For this review, take the finished solid that the model builds, in its own axes (mm). A direction names the side the tool comes from. Give positions to 0.01 mm unless a question says otherwise; leave off trailing zeros. Loops run counter-clockwise (first coordinate to the right, second up) from the corner with the lowest first, then second, coordinate; pieces in that order, holes last. Notation, with made-up numbers: (56.25, 18.5) - (109.25, 18.5) arc R18 cw to (109.25, 38.5) - close; hole circle Ø1 at (54, -10.5). An arc over 180 degrees is marked (long way). Answer in a Markdown table with one row per item.
```python
from build123d import *

# Parameters (mm, degrees)
F0_W      = 30
F0_H      = 43
F1_DEPTH  = 10
F2_W      = 20
F2_H      = 10
F3_DEPTH  = 15
F5_D      = 5.5
F7_D      = 9
F7_DEPTH  = 5
F7_TIP    = 2.7038727856
F8_W      = 20
F8_H      = 43
F9_DEPTH  = 1.55
F11_D     = 3.3
F13_D     = 6
F13_DEPTH = 3
F13_TIP   = 1.8025818571
F14_W     = 6.5
F14_H     = 10
F15_DEPTH = 3.2
F17_D     = 11
F17_DEPTH = 3.5
F17_TIP   = 3.3047334047
F18_R     = 2


with BuildPart() as f1:
    # F0 (on Front) → F1 (new body)
    with BuildSketch(Plane.XZ):
        Rectangle(F0_W, F0_H)
    extrude(amount=F1_DEPTH)

    # F2 (on face) → F3 (join)
    with BuildSketch(Plane.XZ.offset(10)):
        with Locations((0, -16.5)):
            Rectangle(F2_W, F2_H)
    extrude(amount=F3_DEPTH)

    # F5 (through all)
    with Locations(Plane.XY.offset(-11.5)):
        with Locations((0, -17.5)):
            Hole(F5_D / 2)

    # F7
    with Locations(Plane.XY.offset(-11.5)):
        with Locations((0, -17.5)):
            Hole(F7_D / 2, depth=F7_DEPTH)
            with Locations((0, 0, -(F7_DEPTH + F7_TIP / 2))):  # 118° drill point
                Cone(0, F7_D / 2, F7_TIP, mode=Mode.SUBTRACT)

    # F8 (on face) → F9 (cut)
    with BuildSketch(Plane(origin=(0, 0, 0), x_dir=(-1, 0, 0), z_dir=(0, 1, 0))):
        Rectangle(F8_W, F8_H)
    extrude(amount=-F9_DEPTH, mode=Mode.SUBTRACT)

    # F11 (through all)
    with Locations(Plane(origin=(0, -1.55, 0), x_dir=(-1, 0, 0), z_dir=(0, 1, 0))):
        with Locations((0, 1.5)):
            Hole(F11_D / 2)

    # F13
    with Locations(Plane.XZ.offset(10)):
        with Locations((0, 1.5)):
            Hole(F13_D / 2, depth=F13_DEPTH)
            with Locations((0, 0, -(F13_DEPTH + F13_TIP / 2))):  # 118° drill point
                Cone(0, F13_D / 2, F13_TIP, mode=Mode.SUBTRACT)

    # F14 (on face) → F15 (cut)
    with BuildSketch(Plane(origin=(0, -1.55, 0), x_dir=(-1, 0, 0), z_dir=(0, 1, 0))):
        with Locations((-4.25, 16.5)):
            Rectangle(F14_W, F14_H)
        with Locations((-4.25, -16.5)):
            Rectangle(F14_W, F14_H)
    extrude(amount=-F15_DEPTH, mode=Mode.SUBTRACT)

    # F17
    with Locations(Plane(origin=(0, -1.55, 0), x_dir=(-1, 0, 0), z_dir=(0, 1, 0))):
        with Locations((-4.25, -8.5), (-4.25, 11.5)):
            Hole(F17_D / 2, depth=F17_DEPTH)
            with Locations((0, 0, -(F17_DEPTH + F17_TIP / 2))):  # 118° drill point
                Cone(0, F17_D / 2, F17_TIP, mode=Mode.SUBTRACT)

    # F18
    f18_edges = [f1.edges().sort_by_distance(p)[0] for p in [
        (-15, -5, 21.5),
        (0, -10, 21.5),
        (-15, -10, 0),
        (15, -5, 21.5),
        (15, -10, 0),
    ]]
    fillet(f18_edges, radius=F18_R)


solid = f1.part
```
1. We need section D-D, the plane y = -9. Give the boundary of the cut face in (x, z).
Values:
| item | result |
|---|---|
| outline | (-14.73, -21.5) - (14.73, -21.5) - (14.73, 19.5) arc R1.73 ccw to (13, 21.23) - (-13, 21.23) arc R1.73 ccw to (-14.73, 19.5) - close; hole circle Ø6 at (0, 1.5) |
2. Wall thickness on line 1 (X direction, y = -17.5, z = -13.85); line 2 (Z direction, x = 0, y = -3); line 3 (X direction, y = -3, z = 11.5): over which ranges is each line inside the solid? List them lowest first. Write a range as [from, to].
Values:
| item | result |
|---|---|
| line 1 | x = [-10, -4.5], [4.5, 10] |
| line 2 | z = [-21.5, -11.99], [-5.01, -0.15], [3.15, 8.01], [14.99, 21.5] |
| line 3 | x = [-15, -1.25], [9.75, 15] |
3. We need section C-C, the plane x = -7.75. Give the boundary of the cut face in (y, z).
Values:
| item | result |
|---|---|
| outline | (-25, -21.5) - (-1.55, -21.5) - (-1.55, 21.5) - (-8, 21.5) arc R2 ccw to (-10, 19.5) - (-10, -11.5) - (-25, -11.5) - close |
4. Clearance check with flat-ended pins moving along their axes: pin 1 (7 mm diameter, centred on x = 5.5, z = -15.5, fed in from +Y); pin 2 (5 mm diameter, centred on y = -18.5, z = -15, fed in from -X); pin 3 (12 mm diameter, centred on x = -1, z = 3, fed in from +Y); pin 4 (2 mm diameter, centred on x = 0, z = 1.5, fed in from +Y). State where each tip first meets the part, or that it passes through.
Values:
| item | result |
|---|---|
| pin 1 | stops at y = -1.55 |
| pin 2 | stops at x = -10 |
| pin 3 | stops at y = -1.55 |
| pin 4 | passes through |
5. We need section B-B, the plane z = 1.5. Give the boundary of the cut face in (x, y), and give its area (3 significant figures).
Values:
| item | result |
|---|---|
| outline | (-15, -8) arc R2 ccw to (-13, -10) - (-3, -10) - (-3, -7) - (-1.65, -6.19) - (-1.65, -1.55) - (-10, -1.55) - (-10, 0) - (-15, 0) - close; (1.65, -6.19) - (3, -7) - (3, -10) - (13, -10) arc R2 ccw to (15, -8) - (15, 0) - (10, 0) - (10, -1.55) - (1.65, -1.55) - close |
| area | 230 mm^2 |
6. For faces 1 (the face through (-5, -17, -11.5)), 2 (the face through (0.59, -13.04, -14.04)), 3 (the face through (1, -3, -17)), 4 (the face through (10, -1, 0)), list the 3-axis set-ups (+Z, -Z, +X, -X, +Y, -Y) from which the entire face can be reached by the end or side of a thin tool; tool diameter is ignored.
Values:
| item | result |
|---|---|
| face 1 | +Z, +X, -X, -Y |
| face 2 | +Z |
| face 3 | -Z, +Y |
| face 4 | +Z, -Z, +Y |
7. We need section A-A, the plane y = -17.5. Give the boundary of the cut face in (x, z), and give its area (3 significant figures).
Values:
| item | result |
|---|---|
| outline | (-10, -21.5) - (-2.75, -21.5) - (-2.75, -17.55) - (-4.5, -16.5) - (-4.5, -11.5) - (-10, -11.5) - close; (2.75, -21.5) - (10, -21.5) - (10, -11.5) - (4.5, -11.5) - (4.5, -16.5) - (2.75, -17.55) - close |
| area | 126 mm^2 |
8. Mouldability with a two-part tool opening along X and no side actions: class faces 5 (the face through (4, -4.75, 19)), 6 (the face through (10, -17, -17)), 7 (the face through (4, -4.75, -17)), 8 (the face through (-13, 0, 0)) as released by +X, released by -X, zero draft, split by the parting line, or undercut.
Values:
| item | result |
|---|---|
| face 5 | undercut |
| face 6 | released by +X |
| face 7 | undercut |
| face 8 | zero draft |
